Check sheet for the modelled part. Datum: model origin and axes. Units: mm. Face numbers are marked on the shaded views. A direction names the side the tool comes from. Give positions to 0.01 mm unless a question says otherwise; leave off trailing zeros. Write each loop counter-clockwise with the first axis right and the second up, starting at its lowest first coordinate (ties: lowest second). Pieces come first, ordered by that corner, then holes. Notation, with made-up numbers: M -28.75,12.5 L 19.25,12.5 A27 cw 19.25,40.5 Z; hole C 35,33.25 d11. An arc over 180 degrees is marked long. One line per item, written item: value. Start each with the question number.
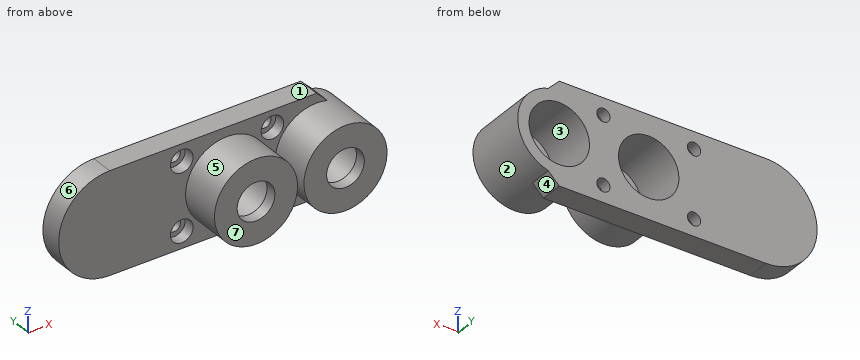
from build123d import *

# Parameters (mm, degrees)
SKETCH1_R               = 1.75
SKETCH1_R_2             = 5
BOSS_EXTRUDE1_DEPTH     = 6
SKETCH2_R               = 3
SKETCH2_R_2             = 1.75
CUT_EXTRUDE1_DEPTH      = 3
CUT_EXTRUDE2_START      = -3
SKETCH3_R               = 8
SKETCH3_R_2             = 5
CUT_EXTRUDE2_DEPTH      = 3
SKETCH5_R               = 13.5
BOSS_EXTRUDE2_DEPTH     = 6
CUT_EXTRUDE3_DEPTH      = 47.983082062
CUT_EXTRUDE3_DEPTH_BACK = 47.983082062
SKETCH6_R               = 8
BOSS_EXTRUDE6_START     = -8
SKETCH9_R               = 11
SKETCH9_R_2             = 8
BOSS_EXTRUDE6_DEPTH     = 8
BOSS_EXTRUDE7_START     = 3
SKETCH10_R              = 11
SKETCH10_R_2            = 5
BOSS_EXTRUDE7_DEPTH     = 3
CHAMFER3_SIZE           = 2.5


with BuildPart() as part:
    # Sketch1 → Boss-Extrude1 (new body)
    with BuildSketch(Plane(origin=(0, 0, 0), x_dir=(1, 0, 0), z_dir=(0, 1, 0))):
        with BuildLine():
            Line((23.69, 13.5), (-31.1, 13.5))
            Line((-31.1, 13.5), (-31.1, 10.5))
            ThreePointArc((-31.1, 10.5), (-20.6, 0), (-31.1, -10.5))
            Line((-31.1, -10.5), (-31.1, -13.5))
            Line((-31.1, -13.5), (23.69, -13.5))
            Line((23.69, -13.5), (23.69, -11))
            ThreePointArc((23.69, -11), (34.69, 0), (23.69, 11))
            Line((23.69, 11), (23.69, 13.5))
        make_face()
        with Locations(Location((-12, -9, 0), (0, 0, 270))):
            Circle(SKETCH1_R, mode=Mode.SUBTRACT)
        with Locations(Location((12, -9, 0), (0, 0, 270))):
            Circle(SKETCH1_R, mode=Mode.SUBTRACT)
        with Locations(Location((-12, 9, 0), (0, 0, 270))):
            Circle(SKETCH1_R, mode=Mode.SUBTRACT)
        with Locations(Location((0, 0, 0), (0, 0, 270))):
            Circle(SKETCH1_R_2, mode=Mode.SUBTRACT)
        with Locations(Location((12, 9, 0), (0, 0, 270))):
            Circle(SKETCH1_R, mode=Mode.SUBTRACT)
        with Locations(Location((23.69, 0, 0), (0, 0, 270))):
            Circle(SKETCH1_R_2, mode=Mode.SUBTRACT)
    extrude(amount=BOSS_EXTRUDE1_DEPTH)

    # Sketch2 → Cut-Extrude1 (cut)
    # profile 1 of 4: a face of its own
    with BuildSketch(Plane.XZ):
        with Locations(Location((-12, -9, 0), (0, 0, 270))):
            Circle(SKETCH2_R)
        with Locations(Location((-12, -9, 0), (0, 0, 270))):
            Circle(SKETCH2_R_2, mode=Mode.SUBTRACT)
    # profile 2 of 4: a face of its own
    with BuildSketch(Plane.XZ):
        with Locations(Location((-12, 9, 0), (0, 0, 270))):
            Circle(SKETCH2_R)
        with Locations(Location((-12, 9, 0), (0, 0, 270))):
            Circle(SKETCH2_R_2, mode=Mode.SUBTRACT)
    # profile 3 of 4: a face of its own
    with BuildSketch(Plane.XZ):
        with Locations(Location((12, 9, 0), (0, 0, 270))):
            Circle(SKETCH2_R)
        with Locations(Location((12, 9, 0), (0, 0, 270))):
            Circle(SKETCH2_R_2, mode=Mode.SUBTRACT)
    # profile 4 of 4: a face of its own
    with BuildSketch(Plane.XZ):
        with Locations(Location((12, -9, 0), (0, 0, 270))):
            Circle(SKETCH2_R)
        with Locations(Location((12, -9, 0), (0, 0, 270))):
            Circle(SKETCH2_R_2, mode=Mode.SUBTRACT)
    extrude(amount=-CUT_EXTRUDE1_DEPTH, mode=Mode.SUBTRACT)

    # Sketch3 → Cut-Extrude2 (cut)
    # profile 1 of 2: a face of its own
    with BuildSketch(Plane(origin=(0, 6, 0), x_dir=(1, 0, 0), z_dir=(0, 1, 0)).offset(CUT_EXTRUDE2_START)):
        with Locations(Location((0, 0, 0), (0, 0, 270))):
            Circle(SKETCH3_R)
        with Locations(Location((0, 0, 0), (0, 0, 270))):
            Circle(SKETCH3_R_2, mode=Mode.SUBTRACT)
    # profile 2 of 2: a face of its own
    with BuildSketch(Plane(origin=(0, 6, 0), x_dir=(1, 0, 0), z_dir=(0, 1, 0)).offset(CUT_EXTRUDE2_START)):
        with Locations(Location((23.69, 0, 0), (0, 0, 270))):
            Circle(SKETCH3_R)
        with Locations(Location((23.69, 0, 0), (0, 0, 270))):
            Circle(SKETCH3_R_2, mode=Mode.SUBTRACT)
    extrude(amount=CUT_EXTRUDE2_DEPTH, mode=Mode.SUBTRACT)

    # Sketch5 → Boss-Extrude2 (add)
    with BuildSketch(Plane(origin=(0, 0, 0), x_dir=(1, 0, 0), z_dir=(0, 1, 0))):
        with Locations((-31.1, 0)):
            Circle(SKETCH5_R)
    extrude(amount=BOSS_EXTRUDE2_DEPTH)

    # Sketch6 → Cut-Extrude3 (cut, two sides: drawn at the far end of the back side and taken through both)
    with BuildSketch(Plane(origin=(0, 6, 0), x_dir=(1, 0, 0), z_dir=(0, 1, 0)).offset(-CUT_EXTRUDE3_DEPTH_BACK)):
        with Locations(Location((0, 0, 0), (0, 0, 270))):
            Circle(SKETCH6_R)
        with Locations(Location((23.69, 0, 0), (0, 0, 270))):
            Circle(SKETCH6_R)
    extrude(amount=CUT_EXTRUDE3_DEPTH + CUT_EXTRUDE3_DEPTH_BACK, mode=Mode.SUBTRACT)

    # Sketch9 → Boss-Extrude6 (add)
    # profile 1 of 2: a face of its own
    with BuildSketch(Plane(origin=(0, 0, 0), x_dir=(1, 0, 0), z_dir=(0, 1, 0)).offset(BOSS_EXTRUDE6_START)):
        with Locations(Location((0, 0, 0), (0, 0, 270))):
            Circle(SKETCH9_R)
        with Locations(Location((0, 0, 0), (0, 0, 270))):
            Circle(SKETCH9_R_2, mode=Mode.SUBTRACT)
    # profile 2 of 2: a face of its own
    with BuildSketch(Plane(origin=(0, 0, 0), x_dir=(1, 0, 0), z_dir=(0, 1, 0)).offset(BOSS_EXTRUDE6_START)):
        with BuildLine():
            ThreePointArc((23.69, 11), (12.69, 0), (23.69, -11))
            ThreePointArc((23.69, -11), (31.468174593, -7.778174593), (34.69, 0))
            ThreePointArc((34.69, 0), (31.468174593, 7.778174593), (23.69, 11))
        make_face()
        with Locations(Location((23.69, 0, 0), (0, 0, 270))):
            Circle(SKETCH9_R_2, mode=Mode.SUBTRACT)
    extrude(amount=BOSS_EXTRUDE6_DEPTH)

    # Sketch10 → Boss-Extrude7 (add)
    # profile 1 of 2: a face of its own
    with BuildSketch(Plane.XZ.offset(8).offset(BOSS_EXTRUDE7_START)):
        with Locations(Location((23.69, 0, 0), (0, 0, 270))):
            Circle(SKETCH10_R)
        with Locations(Location((23.69, 0, 0), (0, 0, 270))):
            Circle(SKETCH10_R_2, mode=Mode.SUBTRACT)
    # profile 2 of 2: a face of its own
    with BuildSketch(Plane.XZ.offset(8).offset(BOSS_EXTRUDE7_START)):
        with Locations(Location((0, 0, 0), (0, 0, 90))):
            Circle(SKETCH10_R)
        with Locations(Location((0, 0, 0), (0, 0, 270))):
            Circle(SKETCH10_R_2, mode=Mode.SUBTRACT)
    extrude(amount=-BOSS_EXTRUDE7_DEPTH)

    # Chamfer3
    # the kernel refuses this chamfer: 2.5 mm, written as the material it adds along each edge
    with BuildSketch(Plane(origin=(23.69, 0, 11), x_dir=(0.9912092295509808, 0, -0.13230367815352337), z_dir=(0, 1, 0))) as chamfer3_piece_1_section:
        with BuildLine():
            Line((2.910680919, 0), (-CHAMFER3_SIZE * 0.132303678154, -CHAMFER3_SIZE * 0.991209229551))
            Line((-CHAMFER3_SIZE * 0.132303678154, -CHAMFER3_SIZE * 0.991209229551), (0, 0))
            ThreePointArc((0, 0), (1.49552658, -0.096625069), (2.910680919, 0))
        make_face()
    chamfer3_piece_1 = extrude(amount=6, mode=Mode.PRIVATE)
    chamfer3_piece_1 = split(chamfer3_piece_1, bisect_by=Plane(origin=(23.69, 0, 13.5), z_dir=(0, 0, -1)), keep=Keep.TOP, mode=Mode.PRIVATE)
    add(chamfer3_piece_1)
    with BuildSketch(Plane(origin=(23.69, 0, -11), x_dir=(0, 0, -1), z_dir=(0, 1, 0))) as chamfer3_piece_2_section:
        with BuildLine():
            Line((CHAMFER3_SIZE, 0), (-0.385093792, -2.885093792))
            ThreePointArc((-0.385093792, -2.885093792), (-0.102088007, -1.495163601), (0, 0))
            Line((0, 0), (CHAMFER3_SIZE, 0))
        make_face()
    chamfer3_piece_2 = extrude(amount=6, mode=Mode.PRIVATE)
    chamfer3_piece_2 = split(chamfer3_piece_2, bisect_by=Plane(origin=(23.69, 0, -13.5), z_dir=(0, 0, 1)), keep=Keep.TOP, mode=Mode.PRIVATE)
    add(chamfer3_piece_2)


solid = part.part
1) Gauge pin test, flat ends, axial feed: pin 1 (3 mm diameter, centred on x = 13, z = 10, fed in from -Y); pin 2 (1.8 mm diameter, centred on x = 12.5, z = -9.5, fed in from -Y); pin 3 (1 mm diameter, centred on x = 25, y = 1, fed in from +Z); pin 4 (2 mm diameter, centred on x = 11, y = -7.5, fed in from -Z). Record the tip position at first contact, or that the pin passes through.
2) Cross-section at D-D (y = -6). Record the boundary of the cut face in (x, z), plus the area to 3 significant figures.
3) Cross-section at A-A (y = 1). Record the boundary of the cut face in (x, z), plus the area to 3 significant figures.
4) Cross-section at B-B (x = 12). Record the boundary of the cut face in (y, z).
5) Tool access check on the marked faces 1, 2 and 3. Record the directions out of +Z, -Z, +X, -X, +Y, -Y that give a thin tool (end or side, any length) a straight path to the whole face; none if there is none.
6) Draft check along X on the marked faces 4, 5, 6 and 7. Enter one of: released by +X, released by -X, zero draft, split by the parting line, or undercut.
7) Cross-section at C-C (z = 2.25). Record the boundary of the cut face in (x, y), plus the area to 3 significant figures.
8) Material ranges on L1, parallel to X at y = -9, z = 0; L2, parallel to X at y = 3.9, z = 9; L3, parallel to X at y = 2.4, z = -9, recorded low to high. Write a range as from..to.
Data:
1. pin 1: stops at y = 3
1. pin 2: passes through
1. pin 3: stops at z = 12.69
1. pin 4: stops at z = -4.58
2. outline: C 0,0 d22; C 23.69,0 d22; hole C 0,0 d16; hole C 23.69,0 d16
2. area: 358 mm2
3. outline: M -31.1,-13.5 L 23.69,-13.5 L 26.58,-10.61 A11 ccw 26.58,10.61 L 23.69,13.5 L -31.1,13.5 A13.5 ccw Z; hole C -12,-9 d6; hole C -12,9 d6; hole C 0,0 d16; hole C 12,-9 d6; hole C 12,9 d6; hole C 23.69,0 d16
3. area: 1,450 mm2
4. outline: M 0,-13.5 L 6,-13.5 L 6,-10.75 L 3,-10.75 L 3,-12 L 0,-12 Z; M 0,-6 L 3,-6 L 3,-7.25 L 6,-7.25 L 6,7.25 L 3,7.25 L 3,6 L 0,6 Z; M 0,12 L 3,12 L 3,10.75 L 6,10.75 L 6,13.5 L 0,13.5 Z
5. face 1: +Z, +X, -X, +Y, -Y
5. face 2: -Y
5. face 3: +Y
6. face 4: released by +X
6. face 5: undercut
6. face 6: released by -X
6. face 7: zero draft
7. outline: M -44.41,0 L -10.77,0 L -10.77,-11 L -4.47,-11 L -4.47,-8 L -7.68,-8 L -7.68,6 L -44.41,6 Z; M 4.47,-11 L 10.77,-11 L 10.77,0 L 12.92,0 L 12.92,-11 L 19.22,-11 L 19.22,-8 L 16.01,-8 L 16.01,6 L 7.68,6 L 7.68,-8 L 4.47,-8 Z; M 28.16,-11 L 34.46,-11 L 34.46,6 L 31.37,6 L 31.37,-8 L 28.16,-8 Z
7. area: 463 mm2
8. L1: x = -11..-5, 5..11, 12.69..18.69, 28.69..34.69
8. L2: x = -41.16..-13.75, -10.25..10.25, 13.75..30.01
8. L3: x = -41.16..-15, -9..9, 15..30.01
